Input: part model. Units: mm. Frame: model coordinates. Face numbers are marked on the shaded views. A direction names the side the tool comes from. Coordinates: 2 decimals unless noted, no trailing zeros. Order: outer loops, then holes, each group sorted by start corner. A loop starts at its lowest first (then second) coordinate and runs counter-clockwise, first axis right, second up. Notation, with made-up numbers: (88, 19) -> (120, 19) arc R12 ccw to (120, 37) -> close; hole circle Ø6 at (37.25, 9). An arc over 180 degrees is marked (long way). One line per question, with ' | ' between items.
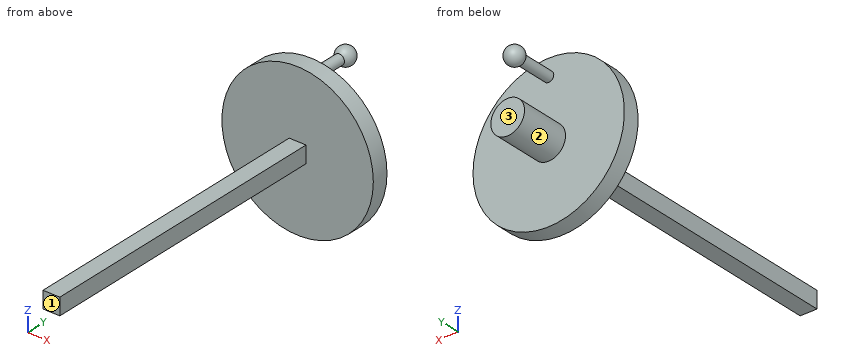
```python
from build123d import *

# Parameters (mm, degrees)
F0_R     = 57.15
F1_DEPTH = 12.7
F2_W     = 12.7
F2_H     = 12.7
F3_DEPTH = 228.6
F4_R     = 12.7
F5_DEPTH = 38.1
F6_R     = 3.81
F7_DEPTH = 31.75


with BuildPart() as f1:
    # F0 (on Front) → F1 (new body)
    with BuildSketch(Plane.XZ):
        Circle(F0_R)
    extrude(amount=F1_DEPTH)

    # F2 (on face) → F3 (join)
    with BuildSketch(Plane.XZ.offset(12.7)):
        Rectangle(F2_W, F2_H)
    extrude(amount=F3_DEPTH)

    # F4 (on face) → F5 (join)
    with BuildSketch(Plane(origin=(0, 0, 0), x_dir=(-1, 0, 0), z_dir=(0, 1, 0))):
        Circle(F4_R)
    extrude(amount=F5_DEPTH)

    # F6 (on face) → F7 (join)
    with BuildSketch(Plane(origin=(0, 0, 0), x_dir=(-1, 0, 0), z_dir=(0, 1, 0))):
        with Locations((0, 44.45)):
            Circle(F6_R)
    extrude(amount=F7_DEPTH)

    # F8 (on face) → F9 (revolve)
    with BuildSketch(Plane(origin=(0, 31.75, 0), x_dir=(-1, 0, 0), z_dir=(0, 1, 0))):
        with BuildLine():
            ThreePointArc((-3.81, 44.45), (0, 48.26), (3.81, 44.45))
            Line((3.81, 44.45), (6.8118199706, 44.45))
            ThreePointArc((6.8118199706, 44.45), (0, 51.2618199706), (-6.8118199706, 44.45))
            Line((-6.8118199706, 44.45), (-3.81, 44.45))
        make_face()
        with BuildLine():
            Line((-3.81, 44.45), (3.81, 44.45))
            ThreePointArc((3.81, 44.45), (0, 48.26), (-3.81, 44.45))
        make_face()
    revolve(axis=Axis((15.5152343214, 31.75, 44.45), (1, 0, 0)))


solid = f1.part
```
1. Ray query, line 1 (X direction, y = -143, z = -4); line 2 (Y direction, x = 3, z = -44). Return the intervals inside material, ascending. Write a range as [from, to].
Recorded:
line 1: x = [-6.35, 6.35] | line 2: y = [-12.7, 0]
2. Cut plane B-B, the plane z = 0. Return loops of the section in (x, y).
Recorded:
outline: (-57.15, -12.7) -> (-6.35, -12.7) -> (-6.35, -241.3) -> (6.35, -241.3) -> (6.35, -12.7) -> (57.15, -12.7) -> (57.15, 0) -> (12.7, 0) -> (12.7, 38.1) -> (-12.7, 38.1) -> (-12.7, 0) -> (-57.15, 0) -> close
3. Access query for the marked faces 1, 2 and 3. Directions: +Z, -Z, +X, -X, +Y, -Y. A direction counts if a zero-diameter tool reaches every point of the face in a straight line with its end or side. Return the directions, or none.
Recorded:
face 1: +Z, -Z, +X, -X, -Y | face 2: +Y | face 3: -Z, +X, -X, +Y
4. Cut plane D-D, the plane z = 44.45. Return loops of the section in (x, y).
Recorded:
outline: (-35.92, -12.7) -> (35.92, -12.7) -> (35.92, 0) -> (3.81, 0) -> (3.81, 26.1) arc R6.81 ccw (long way) to (-3.81, 26.1) -> (-3.81, 0) -> (-35.92, 0) -> close
5. Cut plane A-A, the plane x = 0. Return loops of the section in (y, z).
Recorded:
outline: (-241.3, -6.35) -> (-12.7, -6.35) -> (-12.7, -57.15) -> (0, -57.15) -> (0, -12.7) -> (38.1, -12.7) -> (38.1, 12.7) -> (0, 12.7) -> (0, 40.64) -> (26.1, 40.64) arc R6.81 ccw (long way) to (26.1, 48.26) -> (0, 48.26) -> (0, 57.15) -> (-12.7, 57.15) -> (-12.7, 6.35) -> (-241.3, 6.35) -> close
6. Cut plane C-C, the plane y = -209. Return loops of the section in (x, z), and give its area (3 significant figures).
Recorded:
outline: (-6.35, -6.35) -> (6.35, -6.35) -> (6.35, 6.35) -> (-6.35, 6.35) -> close | area: 161 mm^2
7. Pin query (flat end, axial travel): pin 1 Ø4 at (x, z) = (29.5, -44) entering from -Y; pin 2 Ø10 at (x, y) = (-2.5, -102) entering from +Z; pin 3 Ø7.5 at (x, z) = (-1, 5.5) entering from +Y. Return the tip coordinate at first contact, or that it passes through.
Recorded:
pin 1: stops at y = -12.7 | pin 2: stops at z = 6.35 | pin 3: stops at y = 38.1
